```python
from build123d import *

# Parameters (mm, degrees)
SKETCH_1_W          = 15.7
SKETCH_1_H          = 8.4
EXTRUDE_1_DEPTH     = 37.9
EXTRUDE_2_DEPTH     = 8.4
CUT_EXTRUDE_1_DEPTH = 73.041550511
SKETCH_4_W          = 4.3
SKETCH_4_H          = 4
SKETCH_4_W_2        = 4
CUT_EXTRUDE_2_DEPTH = 73.041550511
SKETCH_5_W          = 5.1
SKETCH_5_H          = 3.1
CUT_EXTRUDE_3_DEPTH = 73.041550511


with BuildPart() as part:
    # ｽｹｯﾁ1 → ﾎﾞｽ - 押し出し1 (new body)
    with BuildSketch(Plane(origin=(0, 0, 0), x_dir=(1, 0, 0), z_dir=(0, 1, 0))):
        Rectangle(SKETCH_1_W, SKETCH_1_H)
    extrude(amount=EXTRUDE_1_DEPTH)

    # ｽｹｯﾁ2 → ﾎﾞｽ - 押し出し2 (add)
    with BuildSketch(Plane.XY.offset(4.2)):
        Polygon((-13.05, 37.9), (11.35, 37.9), (-13.05, 70.35), align=None)
    extrude(amount=-EXTRUDE_2_DEPTH)

    # ｽｹｯﾁ3 → ｶｯﾄ - 押し出し1 (cut, through all)
    with BuildSketch(Plane(origin=(0, 0, -4.2), x_dir=(-1, 0, 0), z_dir=(0, 0, -1))):
        Polygon((10.05, 61.368438838), (-2.610871129, 44.530518012), (10.05, 50.772247606), align=None)
        Polygon((-5.340752161, 40.9), (10.05, 40.9), (10.05, 48.487543721), align=None)
    extrude(amount=-CUT_EXTRUDE_1_DEPTH, mode=Mode.SUBTRACT)

    # ｽｹｯﾁ4 → ｶｯﾄ - 押し出し2 (cut, through all)
    with BuildSketch(Plane(origin=(0, 0, -4.2), x_dir=(-1, 0, 0), z_dir=(0, 0, -1))):
        with Locations((5.7, 2)):
            Rectangle(SKETCH_4_W, SKETCH_4_H)
        with Locations((-5.85, 2)):
            Rectangle(SKETCH_4_W_2, SKETCH_4_H)
    extrude(amount=-CUT_EXTRUDE_2_DEPTH, mode=Mode.SUBTRACT)

    # ｽｹｯﾁ5 → ｶｯﾄ - 押し出し3 (cut, through all)
    with BuildSketch(Plane(origin=(0, 0, -4.2), x_dir=(-1, 0, 0), z_dir=(0, 0, -1))):
        with Locations((3.3, 33.04)):
            Rectangle(SKETCH_5_W, SKETCH_5_H)
    extrude(amount=-CUT_EXTRUDE_3_DEPTH, mode=Mode.SUBTRACT)


solid = part.part
```
Build history of the part. All positions in model axes, mm. A direction names the side the tool comes from. Give positions to 0.01 mm unless a question says otherwise; leave off trailing zeros. Order: outer loops, then holes, each group sorted by start corner. A loop starts at its lowest first (then second) coordinate and runs counter-clockwise, first axis right, second up. Notation, with made-up numbers: M 3.5,85.5 L 29.5,85.5 A23 cw 29.5,94.5 Z; hole C 6.5,-24 d6. An arc over 180 degrees is marked long. Write item = value, one per line. Start each with the question number.
(1) Slice it at B-B on y = 54.5. Write the cut outline in (x, z), plus the area to 3 significant figures.
(2) Probe L1, parallel to Y at x = -5, z = 0.25; L2, parallel to Y at x = -6.5, z = -3.25; L3, parallel to Y at x = -8.5, z = 3. List the from-to ranges inside material, lowest first. Write a range as [from, to].
(3) Slice it at D-D on x = 0.25. Write the cut outline in (y, z), plus the area to 3 significant figures.
(4) Two-plate mould, pull along Y, no slides. Class faces 4 (the flat face through (-6, 4, 0)), 5 (the flat face through (-7.85, 21, 0)), 6 (the flat face through (-2, 40.9, 0)): released by +Y, released by -Y, zero draft, split by the parting line, or undercut.
(5) Pin check, flat tips, straight feed: pin 1 Ø4 at (y, z) = (20.5, -2.5) entering from +X; pin 2 Ø2.5 at (y, z) = (57.5, 0) entering from +X; pin 3 Ø1 at (x, y) = (2, 50.5) entering from +Z; pin 4 Ø1.5 at (y, z) = (33.5, 0) entering from -X. Stop position of each tip, or through.
(6) Slice it at C-C on x = -4.5. Write the cut outline in (y, z).
(7) Slice it at A-A on z = 0. Write the cut outline in (x, y).
(8) Which spindle directions (+Z, -Z, +X, -X, +Y, -Y) get a long thin tool onto all of the face, cutting with end or side? Do faces 1 (the flat face through (0, 0, 0)), 2 (the flat face through (-10.05, 56, 0)), 3 (the flat face through (6, 4, 0)). Say none if no direction does.
Responses:
q1.outline = M -13.05,-4.2 L -10.05,-4.2 L -10.05,4.2 L -13.05,4.2 Z; M -4.89,-4.2 L -1.13,-4.2 L -1.13,4.2 L -4.89,4.2 Z
q1.area = 56.7 mm2
q2.L1 = [4, 31.49], [34.59, 40.9], [46, 48.28], [54.65, 59.64]
q2.L2 = [4, 40.9], [46.74, 49.02], [56.65, 61.64]
q2.L3 = [37.9, 40.9], [47.72, 50.01], [59.31, 64.3]
q3.outline = M 0,-4.2 L 40.9,-4.2 L 40.9,4.2 L 0,4.2 Z; M 43.41,-4.2 L 45.69,-4.2 L 45.69,4.2 L 43.41,4.2 Z; M 47.67,-4.2 L 52.66,-4.2 L 52.66,4.2 L 47.67,4.2 Z
q3.area = 405 mm2
q4.face_4 = released by -Y
q4.face_5 = zero draft
q4.face_6 = undercut
q5.pin_1 = 7.85
q5.pin_2 = -2.45
q5.pin_3 = 4.2
q5.pin_4 = -7.85
q6.outline = M 4,-4.2 L 31.49,-4.2 L 31.49,4.2 L 4,4.2 Z; M 34.59,-4.2 L 40.9,-4.2 L 40.9,4.2 L 34.59,4.2 Z; M 45.75,-4.2 L 48.04,-4.2 L 48.04,4.2 L 45.75,4.2 Z; M 53.99,-4.2 L 58.98,-4.2 L 58.98,4.2 L 53.99,4.2 Z
q7.outline = M -13.05,37.9 L -7.85,37.9 L -7.85,4 L -3.55,4 L -3.55,0 L 3.85,0 L 3.85,4 L 7.85,4 L 7.85,37.9 L 11.35,37.9 L -13.05,70.35 Z; hole M -10.05,40.9 L 5.34,40.9 L -10.05,48.49 Z; hole M -10.05,50.77 L 2.61,44.53 L -10.05,61.37 Z; hole M -5.85,31.49 L -0.75,31.49 L -0.75,34.59 L -5.85,34.59 Z
q8.face_1 = +Z, -Z, +X, -X, -Y
q8.face_2 = +Z, -Z
q8.face_3 = +Z, -Z, +X, -Y
